Geometry: see drawing. Coordinates: mm, zero at the bounding-box minimum. Round coordinates to 2 decimals unless told otherwise and drop trailing zeros. Loops run counter-clockwise (first coordinate to the right, second up) from the corner with the lowest first, then second, coordinate; pieces in that order, holes last. Notation, with made-up numbers: (4, 60) - (33, 60) arc R8 ccw to (33, 74) - close; hole circle Ø2 at (-7.5, 61). An arc over 180 degrees is marked (long way). One line per question, with ' | ' between items. Start each with the question number.
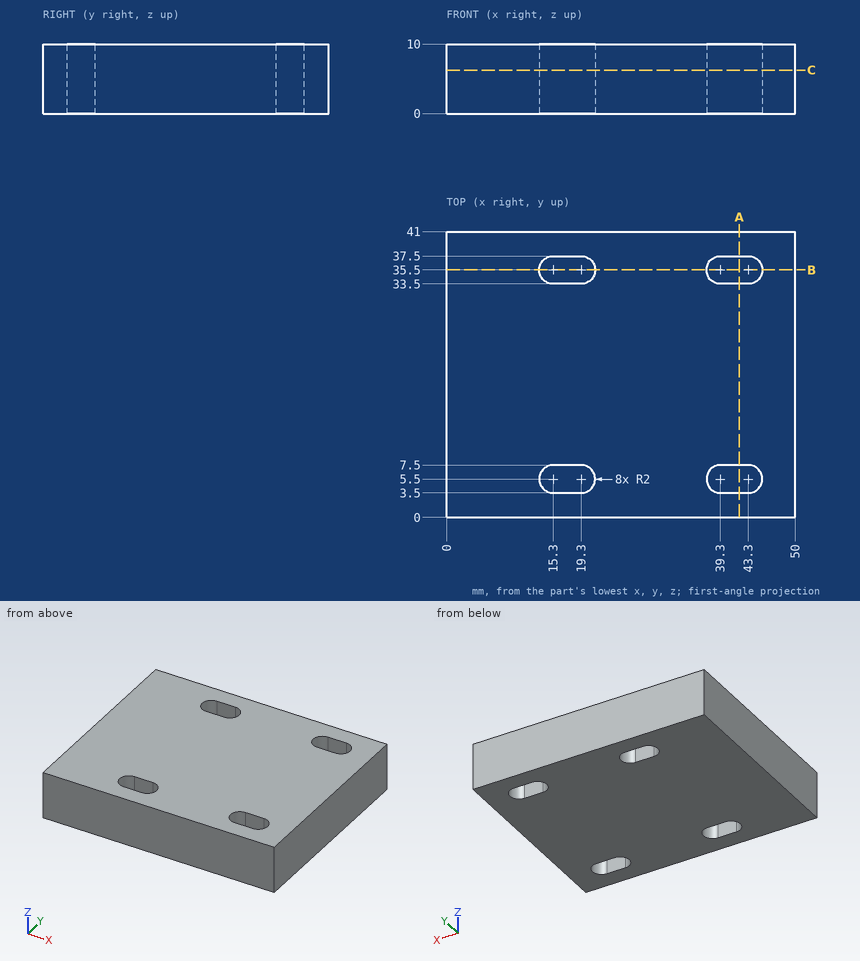
(1) Line query: line 1 along Y through (x, z) = (19, 8.75); line 2 along Y through (x, z) = (20, 8); line 3 along X through (y, z) = (34, 9.25). Output: solid intervals per line, ascending. Write a range as from..to.
(2) Section A-A, the plane x = 42. Output: boundary loops of the cut face in (y, z), plus the area to 3 significant figures.
(3) Section C-C, the plane z = 6.25. Output: boundary loops of the cut face in (x, y), plus the area to 3 significant figures.
(4) Section B-B, the plane y = 35.5. Output: boundary loops of the cut face in (x, z), plus the area to 3 significant figures.
Derived:
1) line 1: y = 0..3.5, 7.5..33.5, 37.5..41 | line 2: y = 0..3.63, 7.37..33.63, 37.37..41 | line 3: x = 0..13.98, 20.62..37.98, 44.62..50
2) outline: (0, 0) - (3.5, 0) - (3.5, 10) - (0, 10) - close; (7.5, 0) - (33.5, 0) - (33.5, 10) - (7.5, 10) - close; (37.5, 0) - (41, 0) - (41, 10) - (37.5, 10) - close | area: 330 mm²
3) outline: (0, 0) - (50, 0) - (50, 41) - (0, 41) - close; hole (15.3, 3.5) - (19.3, 3.5) arc R2 ccw to (19.3, 7.5) - (15.3, 7.5) arc R2 ccw to start; hole (15.3, 33.5) - (19.3, 33.5) arc R2 ccw to (19.3, 37.5) - (15.3, 37.5) arc R2 ccw to start; hole (39.3, 3.5) - (43.3, 3.5) arc R2 ccw to (43.3, 7.5) - (39.3, 7.5) arc R2 ccw to start; hole (39.3, 33.5) - (43.3, 33.5) arc R2 ccw to (43.3, 37.5) - (39.3, 37.5) arc R2 ccw to start | area: 1,940 mm²
4) outline: (0, 0) - (13.3, 0) - (13.3, 10) - (0, 10) - close; (21.3, 0) - (37.3, 0) - (37.3, 10) - (21.3, 10) - close; (45.3, 0) - (50, 0) - (50, 10) - (45.3, 10) - close | area: 340 mm²
